Source: CAD feature listing. Evaluate the final solid. Frame: model axes, mm. Round coordinates to 2 decimals unless told otherwise and drop trailing zeros. Order: outer loops, then holes, each group sorted by start corner. A loop starts at its lowest first (then second) coordinate and runs counter-clockwise, first axis right, second up. Notation, with made-up numbers: (45.25, 5) -> (66.25, 5) arc R18 ccw to (66.25, 33) -> close; hole circle Ø2 at (66, 49.5). An arc over 180 degrees is marked (long way). Answer as CSV lines item,"result". Start each with the question number.
(1) Section query B-B (z = -30). Output: boundary loops of the cut face in (x, y), plus the area to 3 significant figures.
(2) Line query: line 1 along Z through (x, y) = (1.5, 3); line 2 along Z through (x, y) = (0.4, 4.15); line 3 along Z through (x, y) = (-0.9, 1.6). Output: solid intervals per line, ascending. Write a range as from..to.
(3) Section query A-A (x = 0). Output: boundary loops of the cut face in (y, z), plus the area to 3 significant figures.
(4) Pull-direction query (Y, two-part tool) for faces 1 (the cylindrical face through (0, 3, -1)), 2 (the cylindrical face through (0, 3, -29)), 3 (the flat face through (1.2, 6, 0.5)); classes: +Y half, -Y half, draft (parallel to the pull), parting line (faces both ways), or undercut.
(5) Contact query for a flat-ended pin moving along its axis: P1, Ø1.2, axis at x = 0, z = 0, coming from the -Y side. Output: stop coordinate, or through.
(6) Section query C-C (y = 3). Output: boundary loops of the cut face in (x, z), plus the area to 3 significant figures.
(7) Section query D-D (z = -22). Output: boundary loops of the cut face in (x, y), plus the area to 3 significant figures.
```python
from build123d import *

# Parameters (mm, degrees)
SKETCH_1_W          = 5.6
SKETCH_1_H          = 6
EXTRUDE_1_DEPTH     = 34
CUT_EXTRUDE_3_REACH = 36.639
SKETCH_4_R          = 1
CUT_EXTRUDE_4_REACH = 36.977
SKETCH_5_R          = 1


with BuildPart() as part:
    # 草图1 → 凸台-拉伸1 (new, symmetric)
    with BuildSketch(Plane.XY):
        with Locations((0, 3)):
            Rectangle(SKETCH_1_W, SKETCH_1_H)
    extrude(amount=EXTRUDE_1_DEPTH, both=True)

    # 草图4 → 切除-拉伸3 (cut, up to next)
    with BuildSketch(Plane.XZ, mode=Mode.PRIVATE) as cut_extrude_3_sk1:
        Circle(SKETCH_4_R)
    cut_extrude_3_tool1 = extrude(cut_extrude_3_sk1.sketch, amount=-CUT_EXTRUDE_3_REACH, mode=Mode.PRIVATE) & part.part
    # 草图4 → 切除-拉伸3 (cut, up to next)
    with BuildSketch(Plane.XZ, mode=Mode.PRIVATE) as cut_extrude_3_sk2:
        with Locations((0, 22)):
            Circle(SKETCH_4_R)
    cut_extrude_3_tool2 = extrude(cut_extrude_3_sk2.sketch, amount=-CUT_EXTRUDE_3_REACH, mode=Mode.PRIVATE) & part.part
    # 草图4 → 切除-拉伸3 (cut, up to next)
    with BuildSketch(Plane.XZ, mode=Mode.PRIVATE) as cut_extrude_3_sk3:
        with Locations((0, -22)):
            Circle(SKETCH_4_R)
    cut_extrude_3_tool3 = extrude(cut_extrude_3_sk3.sketch, amount=-CUT_EXTRUDE_3_REACH, mode=Mode.PRIVATE) & part.part
    add(cut_extrude_3_tool1.solids().sort_by_distance((0, 0, 0))[0], mode=Mode.SUBTRACT)
    add(cut_extrude_3_tool2.solids().sort_by_distance((0, 0, 22))[0], mode=Mode.SUBTRACT)
    add(cut_extrude_3_tool3.solids().sort_by_distance((0, 0, -22))[0], mode=Mode.SUBTRACT)

    # 草图5 → 切除-拉伸4 (cut, up to next)
    with BuildSketch(Plane(origin=(2.8, 0, 0), x_dir=(0, 0, -1), z_dir=(1, 0, 0)), mode=Mode.PRIVATE) as cut_extrude_4_sk1:
        with Locations(Location((-30, 3, 0), (0, 0, 90))):
            Circle(SKETCH_5_R)
    cut_extrude_4_tool1 = extrude(cut_extrude_4_sk1.sketch, amount=-CUT_EXTRUDE_4_REACH, mode=Mode.PRIVATE) & part.part
    # 草图5 → 切除-拉伸4 (cut, up to next)
    with BuildSketch(Plane(origin=(2.8, 0, 0), x_dir=(0, 0, -1), z_dir=(1, 0, 0)), mode=Mode.PRIVATE) as cut_extrude_4_sk2:
        with Locations(Location((-10, 3, 0), (0, 0, 90))):
            Circle(SKETCH_5_R)
    cut_extrude_4_tool2 = extrude(cut_extrude_4_sk2.sketch, amount=-CUT_EXTRUDE_4_REACH, mode=Mode.PRIVATE) & part.part
    # 草图5 → 切除-拉伸4 (cut, up to next)
    with BuildSketch(Plane(origin=(2.8, 0, 0), x_dir=(0, 0, -1), z_dir=(1, 0, 0)), mode=Mode.PRIVATE) as cut_extrude_4_sk3:
        with Locations(Location((10, 3, 0), (0, 0, 90))):
            Circle(SKETCH_5_R)
    cut_extrude_4_tool3 = extrude(cut_extrude_4_sk3.sketch, amount=-CUT_EXTRUDE_4_REACH, mode=Mode.PRIVATE) & part.part
    # 草图5 → 切除-拉伸4 (cut, up to next)
    with BuildSketch(Plane(origin=(2.8, 0, 0), x_dir=(0, 0, -1), z_dir=(1, 0, 0)), mode=Mode.PRIVATE) as cut_extrude_4_sk4:
        with Locations(Location((30, 3, 0), (0, 0, 90))):
            Circle(SKETCH_5_R)
    cut_extrude_4_tool4 = extrude(cut_extrude_4_sk4.sketch, amount=-CUT_EXTRUDE_4_REACH, mode=Mode.PRIVATE) & part.part
    add(cut_extrude_4_tool1.solids().sort_by_distance((2.8, 3, 30))[0], mode=Mode.SUBTRACT)
    add(cut_extrude_4_tool2.solids().sort_by_distance((2.8, 3, 10))[0], mode=Mode.SUBTRACT)
    add(cut_extrude_4_tool3.solids().sort_by_distance((2.8, 3, -10))[0], mode=Mode.SUBTRACT)
    add(cut_extrude_4_tool4.solids().sort_by_distance((2.8, 3, -30))[0], mode=Mode.SUBTRACT)


solid = part.part
```
Answer block:
1,outline,"(-2.8, 0) -> (2.8, 0) -> (2.8, 2) -> (-2.8, 2) -> close; (-2.8, 4) -> (2.8, 4) -> (2.8, 6) -> (-2.8, 6) -> close"
1,area,"22.4 mm2"
2,line 1,"-34..-31, -29..-11, -9..9, 11..29, 31..34"
2,line 2,"-34..-22.92, -21.08..-0.92, 0.92..21.08, 22.92..34"
2,line 3,"-34..-22.44, -21.56..-0.44, 0.44..21.56, 22.44..34"
3,outline,"(0, -34) -> (6, -34) -> (6, -23) -> (0, -23) -> close; (0, -21) -> (6, -21) -> (6, -1) -> (0, -1) -> close; (0, 1) -> (6, 1) -> (6, 21) -> (0, 21) -> close; (0, 23) -> (6, 23) -> (6, 34) -> (0, 34) -> close; hole circle Ø2 at (3, -30); hole circle Ø2 at (3, -10); hole circle Ø2 at (3, 10); hole circle Ø2 at (3, 30)"
3,area,"359 mm2"
4,face 1,"draft"
4,face 2,"undercut"
4,face 3,"+Y half"
5,P1,"through"
6,outline,"(-2.8, -34) -> (2.8, -34) -> (2.8, -31) -> (-2.8, -31) -> close; (-2.8, -29) -> (2.8, -29) -> (2.8, -11) -> (-2.8, -11) -> close; (-2.8, -9) -> (2.8, -9) -> (2.8, 9) -> (-2.8, 9) -> close; (-2.8, 11) -> (2.8, 11) -> (2.8, 29) -> (-2.8, 29) -> close; (-2.8, 31) -> (2.8, 31) -> (2.8, 34) -> (-2.8, 34) -> close; hole circle Ø2 at (0, -22); hole circle Ø2 at (0, 0); hole circle Ø2 at (0, 22)"
6,area,"327 mm2"
7,outline,"(-2.8, 0) -> (-1, 0) -> (-1, 6) -> (-2.8, 6) -> close; (1, 0) -> (2.8, 0) -> (2.8, 6) -> (1, 6) -> close"
7,area,"21.6 mm2"
